```python
from build123d import *

# Parameters (mm, degrees)
CROQUIS1_R              = 5
SALIENTE_EXTRUIR2_DEPTH = 0.2
CROQUIS2_W              = 2
CROQUIS2_H              = 4.5
SALIENTE_EXTRUIR3_DEPTH = 12.2
CROQUIS7_W              = 4.5
CROQUIS7_H              = 1
SALIENTE_EXTRUIR6_DEPTH = 30
CROQUIS9_R              = 4
SALIENTE_EXTRUIR7_DEPTH = 1
REDONDEO1_R             = 4


with BuildPart() as part:
    # Croquis1 → Saliente-Extruir2 (new body)
    with BuildSketch(Plane(origin=(0, 0, 0), x_dir=(1, 0, 0), z_dir=(0, 1, 0))):
        with BuildLine():
            Line((5.078188303, 2.112345511), (12.443307855, 2.112345511))
            Line((12.443307855, 2.112345511), (12.443307855, -2.387654489))
            Line((12.443307855, -2.387654489), (4.954705444, -2.387654489))
            ThreePointArc((4.954705444, -2.387654489), (-5.49793045, 0.150866705), (5.078188303, 2.112345511))
        make_face()
        Circle(CROQUIS1_R, mode=Mode.SUBTRACT)
    extrude(amount=SALIENTE_EXTRUIR2_DEPTH)

    # Croquis2 → Saliente-Extruir3 (add)
    with BuildSketch(Plane(origin=(0, 0.2, 0), x_dir=(1, 0, 0), z_dir=(0, 1, 0))):
        with Locations((11.443307855, -0.137654489)):
            Rectangle(CROQUIS2_W, CROQUIS2_H)
    extrude(amount=SALIENTE_EXTRUIR3_DEPTH)

    # Croquis7 → Saliente-Extruir6 (add, along a direction that is not the sketch's normal)
    with BuildSketch(Plane(origin=(12.443307855, 0, 0), x_dir=(0, 0, -1), z_dir=(1, 0, 0))):
        with Locations((-0.137654489, 11.9)):
            Rectangle(CROQUIS7_W, CROQUIS7_H)
    extrude(amount=SALIENTE_EXTRUIR6_DEPTH, dir=(0.707106781, 0, -0.707106781))

    # Croquis9 → Saliente-Extruir7 (add)
    with BuildSketch(Plane(origin=(0, 12.4, 0), x_dir=(1, 0, 0), z_dir=(0, 1, 0))):
        with BuildLine():
            Line((33.656511291, 23.325548946), (33.656511291, 18.825548946))
            ThreePointArc((33.656511291, 18.825548946), (45.218660156, 21.075548946), (33.656511291, 23.325548946))
        make_face()
        with Locations((39.218660156, 21.075548946)):
            Circle(CROQUIS9_R, mode=Mode.SUBTRACT)
    extrude(amount=-SALIENTE_EXTRUIR7_DEPTH)

    # Redondeo1
    redondeo1_edges = [part.edges().sort_by_distance(p)[0] for p in [
        (33.656511291, 11.9, -18.825548946),
    ]]
    fillet(redondeo1_edges, radius=REDONDEO1_R)


solid = part.part
```
For this review, take the finished solid that the model builds, in its own axes (mm). A direction names the side the tool comes from. Coordinates: 2 decimals unless noted, no trailing zeros. Loops run counter-clockwise (first coordinate to the right, second up) from the corner with the lowest first, then second, coordinate; pieces in that order, holes last. Notation, with made-up numbers: (42, -18) - (63, -18) arc R16 cw to (63, 3) - close; hole circle Ø11 at (66, -4). An arc over 180 degrees is marked (long way). Use one line per item in the form item = value. Start each with the question number.
1) Take a section at D-D (x = 37.5). State the section outline as (y, z) points, plus the area to 3 significant figures.
2) For faces 4 (the face through (5.5, 0.2, -0.8)), 5 (the face through (22.9, 11.89, -12.57)), list the 3-axis set-ups (+Z, -Z, +X, -X, +Y, -Y) from which the entire face can be reached by the end or side of a thin tool; tool diameter is ignored.
3) Take a section at C-C (z = 1). State the section outline as (x, y) points, plus the area to 3 significant figures.
4) For pin 1 (5 mm diameter, centred on x = 19.5, y = 7, fed in from -Z); pin 2 (14.5 mm diameter, centred on x = 22, z = -7.5, fed in from -Y); pin 3 (10.5 mm diameter, centred on x = 39.22, z = -21.08, fed in from +Y); pin 4 (1.3 mm diameter, centred on y = 8, z = -0.5, fed in from +X), all flat-tipped, find the tip position at first contact; note any pin that passes through.
5) To check wall thickness, follow probe 1 along X at (y, z) = (0.1, 0); probe 2 along Z at (x, y) = (0, 0.15); probe 3 along Y at (x, z) = (17, -4.5). State the ranges of each line that lie inside material, in increasing order. Write a range as from..to.
6) Take a section at B-B (z = -3.5). State the section outline as (x, y) points, plus the area to 3 significant figures.
7) Take a section at A-A (x = 0). State the section outline as (y, z) points, plus the area to 3 significant figures.
8) Draft analysis for pull direction X (two halves, no side actions). For faces 1 (the face through (29, 11.4, -15)), 2 (the face through (33.12, 11.91, -16.92)), 3 (the face through (12.443, 6, 0)), state which applies: released by +X, released by -X, zero draft, split by the parting line, or undercut.
From the geometry:
q1.outline = (11.4, -26.82) - (12.4, -26.82) - (12.4, -24.69) - (11.4, -24.69) - close; (11.4, -17.46) - (12.4, -17.46) - (12.4, -15.33) - (11.4, -15.33) - close
q1.area = 4.27 mm2
q2.face_4 = +Z, -Z, -X, +Y
q2.face_5 = -Z, -X, +Y, -Y
q3.outline = (-5.41, 0) - (-4.9, 0) - (-4.9, 0.2) - (-5.41, 0.2) - close; (4.9, 0) - (12.44, 0) - (12.44, 11.4) - (13.83, 11.4) - (13.83, 12.4) - (10.44, 12.4) - (10.44, 0.2) - (4.9, 0.2) - close
q3.area = 27.4 mm2
q4.pin_1 = through
q4.pin_2 = 11.4
q4.pin_3 = 12.4
q4.pin_4 = 12.44
q5.probe_1 = -5.5..-5, 5..12.44
q5.probe_2 = -5.5..-5, 5..5.5
q5.probe_3 = 11.4..12.4
q6.outline = (-4.24, 0) - (-3.57, 0) - (-3.57, 0.2) - (-4.24, 0.2) - close; (3.57, 0) - (4.24, 0) - (4.24, 0.2) - (3.57, 0.2) - close; (13.83, 11.4) - (18.33, 11.4) - (18.33, 12.4) - (13.83, 12.4) - close
q6.area = 4.77 mm2
q7.outline = (0, -5.5) - (0.2, -5.5) - (0.2, -5) - (0, -5) - close; (0, 5) - (0.2, 5) - (0.2, 5.5) - (0, 5.5) - close
q7.area = 0.200 mm2
q8.face_1 = zero draft
q8.face_2 = undercut
q8.face_3 = released by +X
